Verification items for this drawing (mm, ordinates from the low corner). Give positions to 0.01 mm unless a question says otherwise; leave off trailing zeros. Write each loop counter-clockwise with the first axis right and the second up, starting at its lowest first coordinate (ties: lowest second). Pieces come first, ordered by that corner, then holes. Notation, with made-up numbers: (15, -15.75) -> (45, -15.75) arc R9 ccw to (45, 0.25) -> close; hole circle Ø11 at (5, 6). An arc over 180 degrees is marked (long way). Answer as a JSON object with one key per item and string values.
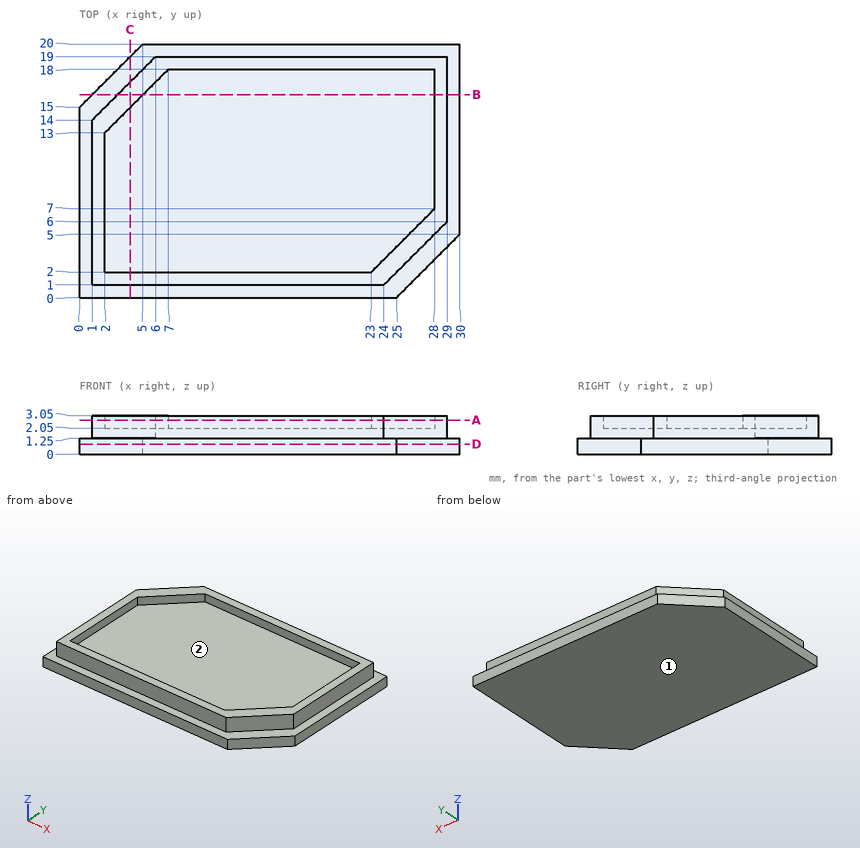
1. Sectioned sample at A-A, the plane z = 2.7. Enter the section's corners in (x, y).
Determined:
{"outline": "(1, 1) -> (24, 1) -> (29, 6) -> (29, 19) -> (6, 19) -> (1, 14) -> close; hole (2, 2) -> (23, 2) -> (28, 7) -> (28, 18) -> (7, 18) -> (2, 13) -> close"}
2. Sectioned sample at B-B, the plane y = 16. Enter the section's corners in (x, z), plus the area to 4 significant figures.
Determined:
{"outline": "(1, 0) -> (30, 0) -> (30, 1.25) -> (29, 1.25) -> (29, 3.05) -> (28, 3.05) -> (28, 2.05) -> (5, 2.05) -> (5, 3.05) -> (3, 3.05) -> (3, 1.25) -> (1, 1.25) -> close", "area": "60.05 mm^2"}
3. Sectioned sample at D-D, the plane z = 0.8. Enter the section's corners in (x, y).
Determined:
{"outline": "(0, 0) -> (25, 0) -> (30, 5) -> (30, 20) -> (5, 20) -> (0, 15) -> close"}
4. Mould release check, pull along Y, two halves, no side actions. Record for the marked faces 1 and 2: released by +Y, released by -Y, zero draft, split by the parting line, or undercut.
Determined:
{"face 1": "zero draft", "face 2": "undercut"}
5. Go/stop test with flat-tipped pins: P1, Ø1.5, axis at x = 5, y = 9, coming from the +Z side; P2, Ø0.9, axis at x = 11.5, z = 1.5, coming from the -Y side; P3, Ø0.5, axis at x = 10.5, z = 2.5, coming from the +Y side; P4, Ø0.8, axis at y = 9.5, z = 3, coming from the +X side. Record where each tip stops, or that it passes through.
Determined:
{"P1": "z = 2.05", "P2": "y = 0", "P3": "y = 19", "P4": "x = 29"}
6. Scan lines: L1, parallel to Y at x = 19.25, z = 2.75; L2, parallel to Z at x = 21.75, y = 15.5; L3, parallel to X at y = 4.25, z = 2.95. Record each from-to range of solid material in increasing order. Write a range as [from, to].
Determined:
{"L1": "[1, 2], [18, 19]", "L2": "[0, 2.05]", "L3": "[1, 2], [25.25, 27.25]"}
7. Sectioned sample at C-C, the plane x = 4. Enter the section's corners in (y, z), plus the area to 4 significant figures.
Determined:
{"outline": "(0, 0) -> (19, 0) -> (19, 1.25) -> (17, 1.25) -> (17, 3.05) -> (15, 3.05) -> (15, 2.05) -> (2, 2.05) -> (2, 3.05) -> (1, 3.05) -> (1, 1.25) -> (0, 1.25) -> close", "area": "39.55 mm^2"}
